Read the model definition and answer for the solid it produces. Units are mm, in the model's axes. A direction names the side the tool comes from. Coordinates: 2 decimals unless noted, no trailing zeros. Loops run counter-clockwise (first coordinate to the right, second up) from the corner with the lowest first, then second, coordinate; pieces in that order, holes last. Notation, with made-up numbers: (70, -24.5) -> (82, -24.5) arc R19 ccw to (82, -0.5) -> close; hole circle Ø10 at (39.5, 32.5). An arc over 180 degrees is marked (long way). Answer as a JSON object with one key per item and string values. Group by question number.
Q1. A straight line is drawn through the part: line 1 along Y through (x, z) = (121, -11.5). Find the intervals that lie inside material, in ascending order. Write a range as [from, to].
Q2. Determine the mould class of faces 5 (the flat face through (65, 110.25, -5)), 6 (the flat face through (127, 116, -5)), 7 (the flat face through (122, 97.25, -5)) for opening direction Y: released by +Y, released by -Y, zero draft, split by the parting line, or undercut.
Q3. The part is cut by section B-B on y = 106. Write down the section's boundary in (x, z), and give its area (3 significant figures).
Q4. For faces 1 (the flat face through (102, 97.25, -5)), 2 (the flat face through (65, 97.25, -5)), 3 (the flat face through (131, 110.75, -5)), 4 (the flat face through (122, 110.75, -5)), determine the directions among +Z, -Z, +X, -X, +Y, -Y from which every point of the face is accessible in a straight line to the end or side of a thin tool.
Q5. Each of these flat-tipped pins is pushed along its axis until it touches: P1, Ø0.6, axis at x = 65.5, z = -7, coming from the +Y side; P2, Ø1, axis at y = 104, z = 2.5, coming from the +X side; P3, Ø7.5, axis at x = 92.5, z = -6.5, coming from the -Y side. Where does it stop, or does it pass through?
Q6. The part is cut by section C-C on z = -19. State how many separate pieces and enclosed holes the cut face has, and give its area (3 significant figures).
Q7. The part is cut by section A-A on x = 113. Write down the section's boundary in (y, z).
from build123d import *

# Parameters (mm, degrees)
BOX029_W     = 0.5
BOX029_H     = 36.5
BOX029_DEPTH = 36.8
BOX030_W     = 0.5
BOX030_H     = 36.5
BOX030_DEPTH = 36.8
BOX034_W     = 71.5
BOX034_H     = 0.5
BOX034_DEPTH = 36.8
BOX032_W     = 0.5
BOX032_H     = 36.5
BOX032_DEPTH = 36.8
BOX028_W     = 0.5
BOX028_H     = 36.5
BOX028_DEPTH = 36.8
BOX027_W     = 0.5
BOX027_H     = 36.5
BOX027_DEPTH = 36.8
BOX031_W     = 0.5
BOX031_H     = 36.5
BOX031_DEPTH = 36.8
BOX033_W     = 71.5
BOX033_H     = 0.5
BOX033_DEPTH = 36.8
BOX026_W     = 0.5
BOX026_H     = 36.5
BOX026_DEPTH = 36.8


with BuildPart() as box029:
    # Box029 → Box029 (new body)
    with BuildSketch(Plane(origin=(96.5, 85.25, -23), x_dir=(1, 0, 0), z_dir=(0, 0, 1))):
        with Locations((0.25, 18.25)):
            Rectangle(BOX029_W, BOX029_H)
    extrude(amount=BOX029_DEPTH)


with BuildPart() as box030:
    # Box030 → Box030 (new body)
    with BuildSketch(Plane(origin=(86.5, 85.25, -23), x_dir=(1, 0, 0), z_dir=(0, 0, 1))):
        with Locations((0.25, 18.25)):
            Rectangle(BOX030_W, BOX030_H)
    extrude(amount=BOX030_DEPTH)


with BuildPart() as box034:
    # Box034 → Box034 (new body)
    with BuildSketch(Plane(origin=(64.5, 110.25, -23), x_dir=(1, 0, 0), z_dir=(0, 0, 1))):
        with Locations((35.75, 0.25)):
            Rectangle(BOX034_W, BOX034_H)
    extrude(amount=BOX034_DEPTH)


with BuildPart() as box032:
    # Box032 → Box032 (new body)
    with BuildSketch(Plane(origin=(66.5, 85.25, -23), x_dir=(1, 0, 0), z_dir=(0, 0, 1))):
        with Locations((0.25, 18.25)):
            Rectangle(BOX032_W, BOX032_H)
    extrude(amount=BOX032_DEPTH)


with BuildPart() as box028:
    # Box028 → Box028 (new body)
    with BuildSketch(Plane(origin=(106.5, 85.25, -23), x_dir=(1, 0, 0), z_dir=(0, 0, 1))):
        with Locations((0.25, 18.25)):
            Rectangle(BOX028_W, BOX028_H)
    extrude(amount=BOX028_DEPTH)


with BuildPart() as box027:
    # Box027 → Box027 (new body)
    with BuildSketch(Plane(origin=(116.5, 85.25, -23), x_dir=(1, 0, 0), z_dir=(0, 0, 1))):
        with Locations((0.25, 18.25)):
            Rectangle(BOX027_W, BOX027_H)
    extrude(amount=BOX027_DEPTH)


with BuildPart() as box031:
    # Box031 → Box031 (new body)
    with BuildSketch(Plane(origin=(76.5, 85.25, -23), x_dir=(1, 0, 0), z_dir=(0, 0, 1))):
        with Locations((0.25, 18.25)):
            Rectangle(BOX031_W, BOX031_H)
    extrude(amount=BOX031_DEPTH)


with BuildPart() as box033:
    # Box033 → Box033 (new body)
    with BuildSketch(Plane(origin=(64.5, 97.25, -23), x_dir=(1, 0, 0), z_dir=(0, 0, 1))):
        with Locations((35.75, 0.25)):
            Rectangle(BOX033_W, BOX033_H)
    extrude(amount=BOX033_DEPTH)


with BuildPart() as support:
    # Box026 → Box026 (new body)
    with BuildSketch(Plane(origin=(126.5, 85.25, -23), x_dir=(1, 0, 0), z_dir=(0, 0, 1))):
        with Locations((0.25, 18.25)):
            Rectangle(BOX026_W, BOX026_H)
    extrude(amount=BOX026_DEPTH)

    # Fusion019: union Box029, Box030, Box034, Box032, Box028, Box027, Box031, Box033
    add(box029.part)
    add(box030.part)
    add(box034.part)
    add(box032.part)
    add(box028.part)
    add(box027.part)
    add(box031.part)
    add(box033.part)


solid = support.part
Final values:
{
 "1": {"line 1": "y = [97.25, 97.75], [110.25, 110.75]"},
 "2": {"face 5": "undercut", "face 6": "zero draft", "face 7": "released by -Y"},
 "3": {"outline": "(66.5, -23) -> (67, -23) -> (67, 13.8) -> (66.5, 13.8) -> close; (76.5, -23) -> (77, -23) -> (77, 13.8) -> (76.5, 13.8) -> close; (86.5, -23) -> (87, -23) -> (87, 13.8) -> (86.5, 13.8) -> close; (96.5, -23) -> (97, -23) -> (97, 13.8) -> (96.5, 13.8) -> close; (106.5, -23) -> (107, -23) -> (107, 13.8) -> (106.5, 13.8) -> close; (116.5, -23) -> (117, -23) -> (117, 13.8) -> (116.5, 13.8) -> close; (126.5, -23) -> (127, -23) -> (127, 13.8) -> (126.5, 13.8) -> close", "area": "129 mm2"},
 "4": {"face 1": "+Z, -Z, -Y", "face 2": "+Z, -Z, -X, -Y", "face 3": "+Z, -Z, +X, +Y", "face 4": "+Z, -Z, +Y"},
 "5": {"P1": "stops at y = 110.75", "P2": "stops at x = 127", "P3": "stops at y = 97.25"},
 "6": {"separate pieces": "1", "enclosed holes": "6", "area": "196 mm2"},
 "7": {"outline": "(97.25, -23) -> (97.75, -23) -> (97.75, 13.8) -> (97.25, 13.8) -> close; (110.25, -23) -> (110.75, -23) -> (110.75, 13.8) -> (110.25, 13.8) -> close"}
}
